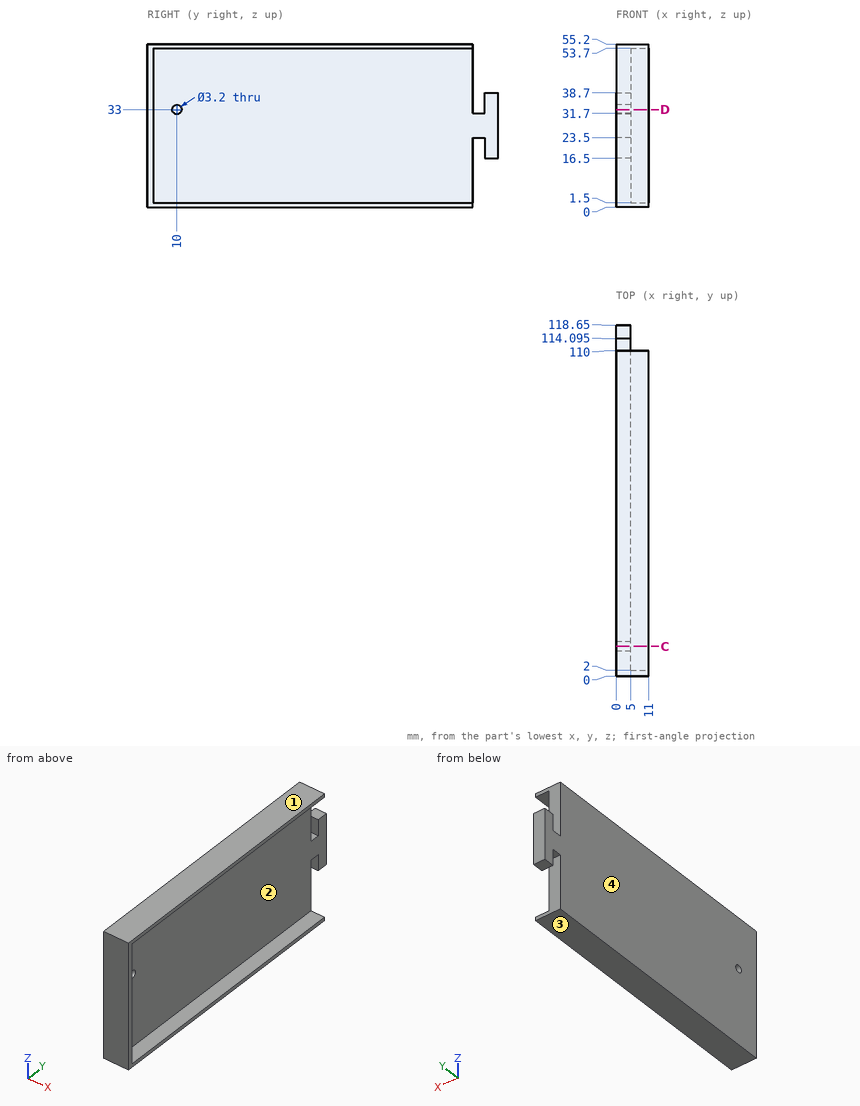
Geometry check sheet. Reference: drawing and pictorial views, mm from the part's lowest x, y, z. Coordinates: 2 decimals unless noted, no trailing zeros. Loops run counter-clockwise (first coordinate to the right, second up) from the corner with the lowest first, then second, coordinate; pieces in that order, holes last. Notation, with made-up numbers: M 28,-13 L 56,-13 A26 ccw 56,24 Z; hole C -8.5,-13 d3. An arc over 180 degrees is marked long. One line per item, written item: value.
1. Gauge pin test, flat ends, axial feed: P1, Ø4, axis at y = 41, z = 27.5, coming from the +X side; P2, Ø1.2, axis at x = 1.5, y = 111.5, coming from the -Z side; P3, Ø3.5, axis at x = 2.5, y = 117, coming from the -Z side. Record the tip position at first contact, or that the pin passes through.
Answers follow:
P1: x = 5
P2: z = 23.5
P3: z = 16.5
2. Material ranges on line 1 along Z through (x, y) = (8.5, 24); line 2 along Z through (x, y) = (2.4, 10); line 3 along X through (y, z) = (20, 14.5), recorded low to high. Write a range as from..to.
Answers follow:
line 1: 0..1.5, 53.7..55.2
line 2: 0..31.4, 34.6..55.2
line 3: 0..5
3. Mould release check, pull along Z, two halves, no side actions. Record for the marked faces 1, 2, 3 and 4: pulls with the +Z half, pulls with the -Z half, needs draft (parallel to the pull), parting line crosses it, or undercut.
Answers follow:
face 1: pulls with the +Z half
face 2: undercut
face 3: pulls with the -Z half
face 4: needs draft
4. Section check D-D on z = 33. Give the number of separate pieces and of enclosed holes in the cut face, plus the area to 3 significant figures.
Answers follow:
separate pieces: 3
enclosed holes: 0
area: 569 mm^2
5. Section check C-C on y = 10. Record the cut outline in (x, z), plus the area to 3 significant figures.
Answers follow:
outline: M 0,0 L 11,0 L 11,1.5 L 5,1.5 L 5,31.4 L 0,31.4 Z; M 0,34.6 L 5,34.6 L 5,53.7 L 11,53.7 L 11,55.2 L 0,55.2 Z
area: 278 mm^2
